Source: CAD feature listing. Evaluate the final solid. Frame: model axes, mm. Coordinates: 2 decimals unless noted, no trailing zeros. Loops run counter-clockwise (first coordinate to the right, second up) from the corner with the lowest first, then second, coordinate; pieces in that order, holes last. Notation, with made-up numbers: (-19, -9) - (6, -9) arc R19 cw to (6, 12) - close; hole circle Ø6 at (-40, 28). An arc over 180 degrees is marked (long way). Use CSV: the item, a comma, the result in double quotes. Start each with the question number.
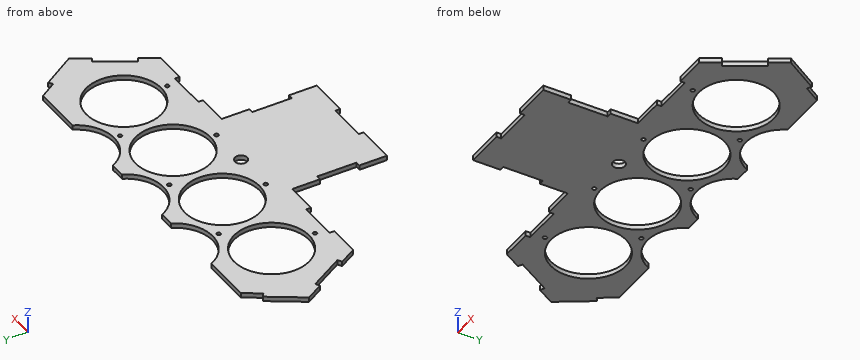
```python
from build123d import *

# Parameters (mm, degrees)
ESQUISSE1_R             = 47.5
BOSS_EXTRU_1_DEPTH      = 6
ESQUISSE9_W             = 150
ESQUISSE9_H             = 120
BOSS_EXTRU_2_DEPTH      = 6
ESQUISSE10_W            = 6
ESQUISSE10_H            = 50
ESQUISSE10_W_2          = 50
ESQUISSE10_H_2          = 6
ENL_V_MAT_EXTRU_1_DEPTH = 10
ESQUISSE12_W            = 675.538278175
ESQUISSE12_H            = 265.771999275
ENL_V_MAT_EXTRU_3_DEPTH = 10
ESQUISSE13_R            = 2.5
ENL_V_MAT_EXTRU_4_DEPTH = 10
ESQUISSE14_R            = 7.75
ENL_V_MAT_EXTRU_5_DEPTH = 10


with BuildPart() as part:
    # Esquisse1 → Boss.-Extru.1 (new body)
    with BuildSketch(Plane.XY):
        Polygon((-255.775862069, 10.959681362), (-205, -75.190256718), (205, -75.190256718), (255.775862069, 10.959681362), (50, 336.353741833), (-50, 336.353741833), align=None)
        with Locations((-157.5, 0)):
            Circle(ESQUISSE1_R, mode=Mode.SUBTRACT)
        with Locations((-52.5, 0)):
            Circle(ESQUISSE1_R, mode=Mode.SUBTRACT)
        with Locations((52.5, 0)):
            Circle(ESQUISSE1_R, mode=Mode.SUBTRACT)
        with Locations((157.5, 0)):
            Circle(ESQUISSE1_R, mode=Mode.SUBTRACT)
        with Locations((-105, 90.932667397)):
            Circle(ESQUISSE1_R, mode=Mode.SUBTRACT)
        with Locations((0, 90.932667397)):
            Circle(ESQUISSE1_R, mode=Mode.SUBTRACT)
        with Locations((105, 90.932667397)):
            Circle(ESQUISSE1_R, mode=Mode.SUBTRACT)
        with Locations((-52.5, 181.865334795)):
            Circle(ESQUISSE1_R, mode=Mode.SUBTRACT)
        with Locations((52.5, 181.865334795)):
            Circle(ESQUISSE1_R, mode=Mode.SUBTRACT)
        with Locations((0, 272.798002192)):
            Circle(ESQUISSE1_R, mode=Mode.SUBTRACT)
    extrude(amount=BOSS_EXTRU_1_DEPTH)

    # Esquisse9 → Boss.-Extru.2 (add)
    with BuildSketch(Plane.XY.offset(6)):
        with Locations((0, -135.190256718)):
            Rectangle(ESQUISSE9_W, ESQUISSE9_H)
    extrude(amount=-BOSS_EXTRU_2_DEPTH)

    # Esquisse10 → Enlèv. mat.-Extru.1 (cut)
    with BuildSketch(Plane.XY.offset(6)):
        with Locations((-72, -135.190256718)):
            Rectangle(ESQUISSE10_W, ESQUISSE10_H)
        with Locations((0, -192.190256718)):
            Rectangle(ESQUISSE10_W_2, ESQUISSE10_H_2)
        with Locations((-140, -72.190256718)):
            Rectangle(ESQUISSE10_W_2, ESQUISSE10_H_2)
        Polygon((-217.693965517, -53.652772198), (-212.524969232, -50.606220473), (-237.912900267, -7.531251434), (-243.081896552, -10.577803158), align=None)
        Polygon((-229.051724138, 53.218650255), (-223.980647871, 50.011753703), (-170.532372009, 134.529691487), (-175.603448276, 137.736588039), align=None)
        Polygon((-130.172413793, 209.576835156), (-125.101337526, 206.369938604), (-71.653061664, 290.887876389), (-76.724137931, 294.094772941), align=None)
        with Locations((0, 333.353741833)):
            Rectangle(ESQUISSE10_W_2, ESQUISSE10_H_2)
        Polygon((71.653061664, 290.887876389), (76.724137931, 294.094772941), (130.172413793, 209.576835156), (125.101337526, 206.369938604), align=None)
        Polygon((170.532372009, 134.529691487), (175.603448276, 137.736588039), (229.051724138, 53.218650255), (223.980647871, 50.011753703), align=None)
        Polygon((237.912900267, -7.531251434), (243.081896552, -10.577803158), (217.693965517, -53.652772198), (212.524969232, -50.606220473), align=None)
        with Locations((140, -72.190256718)):
            Rectangle(ESQUISSE10_W_2, ESQUISSE10_H_2)
        with Locations((72, -135.190256718)):
            Rectangle(ESQUISSE10_W, ESQUISSE10_H)
    extrude(amount=-ENL_V_MAT_EXTRU_1_DEPTH, mode=Mode.SUBTRACT)

    # Esquisse12 → Enlèv. mat.-Extru.3 (cut)
    with BuildSketch(Plane.XY.offset(6)):
        with Locations((-8.823645222, 203.467742196)):
            Rectangle(ESQUISSE12_W, ESQUISSE12_H)
    extrude(amount=-ENL_V_MAT_EXTRU_3_DEPTH, mode=Mode.SUBTRACT)

    # Esquisse13 → Enlèv. mat.-Extru.4 (cut)
    with BuildSketch(Plane.XY.offset(6)):
        with Locations((-157.5, -55)):
            Circle(ESQUISSE13_R)
        with Locations((-52.5, -55)):
            Circle(ESQUISSE13_R)
        with Locations((52.5, -55)):
            Circle(ESQUISSE13_R)
        with Locations((157.5, -55)):
            Circle(ESQUISSE13_R)
        with Locations((-105, 35.932667397)):
            Circle(ESQUISSE13_R)
        with Locations((0, 35.932667397)):
            Circle(ESQUISSE13_R)
        with Locations((105, 35.932667397)):
            Circle(ESQUISSE13_R)
    extrude(amount=-ENL_V_MAT_EXTRU_4_DEPTH, mode=Mode.SUBTRACT)

    # Esquisse14 → Enlèv. mat.-Extru.5 (cut)
    with BuildSketch(Plane.XY.offset(6)):
        with Locations((0, -55)):
            Circle(ESQUISSE14_R)
    extrude(amount=-ENL_V_MAT_EXTRU_5_DEPTH, mode=Mode.SUBTRACT)


solid = part.part
```
(1) Section D-D on x = -173.5. Output: boundary loops of the cut face in (y, z).
(2) Section A-A on x = 15. Output: boundary loops of the cut face in (y, z).
(3) Ray query, line 1 (Y direction, x = 157.5, z = 1.55); line 2 (X direction, y = 11, z = 4.75); line 3 (Y direction, x = 105, z = 4.7). Return the intervals inside material, ascending. Write a range as [from, to].
(4) Pin query (flat end, axial travel): pin 1 Ø3 at (y, z) = (-72, 3.5) entering from -X; pin 2 Ø3 at (x, z) = (91.5, 3.5) entering from -Y; pin 3 Ø1.8 at (y, z) = (-73, 4.5) entering from -X. Return the tip coordinate at first contact, or that it passes through.
(5) Section B-B on y = -24.5. Output: boundary loops of the cut face in (x, z).
(6) Section C-C on y = -143. Output: boundary loops of the cut face in (x, z), plus the area to 3 significant figures.
Solution:
1,outline,"(-75.19, 0) - (-44.72, 0) - (-44.72, 6) - (-75.19, 6) - close; (44.72, 0) - (70.58, 0) - (70.58, 6) - (44.72, 6) - close"
2,outline,"(-189.19, 0) - (-29.15, 0) - (-29.15, 6) - (-189.19, 6) - close; (29.15, 0) - (45.86, 0) - (45.86, 6) - (29.15, 6) - close"
3,line 1,"y = [-69.19, -57.5], [-52.5, -47.5], [47.5, 70.58]"
3,line 2,"x = [-255.75, -203.71], [-111.29, -98.71], [-6.29, 6.29], [98.71, 111.29], [203.71, 255.75]"
3,line 3,"y = [-75.19, 33.43], [38.43, 43.43]"
4,pin 1,"stops at x = -207.76"
4,pin 2,"stops at y = -75.19"
4,pin 3,"stops at x = -206.82"
5,outline,"(-227.91, 0) - (-198.19, 0) - (-198.19, 6) - (-227.91, 6) - close; (-116.81, 0) - (-93.19, 0) - (-93.19, 6) - (-116.81, 6) - close; (-11.81, 0) - (11.81, 0) - (11.81, 6) - (-11.81, 6) - close; (93.19, 0) - (116.81, 0) - (116.81, 6) - (93.19, 6) - close; (198.19, 0) - (227.91, 0) - (227.91, 6) - (198.19, 6) - close"
6,outline,"(-69, 0) - (69, 0) - (69, 6) - (-69, 6) - close"
6,area,"828 mm²"
